Model file for the job. Use its own axes, mm. A direction names the side the tool comes from. Coordinates: 2 decimals unless noted, no trailing zeros. Loops run counter-clockwise (first coordinate to the right, second up) from the corner with the lowest first, then second, coordinate; pieces in that order, holes last. Notation, with made-up numbers: M -0.5,81.5 L 12.5,81.5 A18 cw 12.5,90.5 Z; hole C 60.25,-20.5 d2. An arc over 180 degrees is marked long. Write item = value, one per line. Start each with the question number.
from build123d import *

# Parameters (mm, degrees)
ESQUISSE1_W             = 70
ESQUISSE1_H             = 110
BOSS_EXTRU_1_DEPTH      = 3
ENL_V_MAT_EXTRU_1_DEPTH = 131.418556962
ENL_V_MAT_EXTRU_2_DEPTH = 10


with BuildPart() as part:
    # Esquisse1 → Boss.-Extru.1 (new body)
    with BuildSketch(Plane.XY):
        with Locations((-35, 55)):
            Rectangle(ESQUISSE1_W, ESQUISSE1_H)
    extrude(amount=BOSS_EXTRU_1_DEPTH)

    # Esquisse2 → Enlèv. mat.-Extru.1 (cut, through all)
    with BuildSketch(Plane(origin=(0, 0, 0), x_dir=(-1, 0, 0), z_dir=(0, 0, -1))):
        Polygon((0, 110), (25, 110), (25, 104), (6, 104), (6, 68.5), (0, 68.5), align=None)
        Polygon((70, 110), (45, 110), (45, 104), (64, 104), (64, 68.5), (70, 68.5), align=None)
        Polygon((0, 0), (25, 0), (25, 6), (6, 6), (6, 38.5), (0, 38.5), align=None)
        Polygon((45, 0), (70, 0), (70, 38.5), (64, 38.5), (64, 6), (45, 6), align=None)
    extrude(amount=-ENL_V_MAT_EXTRU_1_DEPTH, mode=Mode.SUBTRACT)

    # Esquisse3 → Enlèv. mat.-Extru.2 (cut)
    with BuildSketch(Plane.XY.offset(3)):
        Polygon((-70, 38.5), (-25, 38.5), (-25, 81.225715449), (-2.235916109, 81.225715449), (-2.235916109, 110), (-25, 110), (-70, 110), align=None)
    extrude(amount=-ENL_V_MAT_EXTRU_2_DEPTH, mode=Mode.SUBTRACT)


solid = part.part
Item 1: Cut at C-C (y = 43.5). Give the cut face in (x, z).
Item 2: 3-axis set-ups, long thin cutter, end or side, ignore diameter. For faces 1 (the flat face through (-45, 38.5, 2)), 2 (the flat face through (-3, 68.5, 1)), 3 (the flat face through (-45, 3, 1)): which of +Z, -Z, +X, -X, +Y, -Y reach the whole face in a straight line?
Item 3: Pin check, flat tips, straight feed: pin 1 Ø1.5 at (y, z) = (17, 1) entering from +X; pin 2 Ø1.5 at (y, z) = (63, 1) entering from +X; pin 3 Ø0.9 at (x, z) = (-11, 1) entering from -Y; pin 4 Ø0.9 at (x, z) = (-51.5, 1.5) entering from +Y. Stop position of each tip, or through.
Item 4: Cut at A-A (z = 1.1). Give the cut face in (x, y), plus the area to 3 significant figures.
Item 5: Cut at B-B (x = -53.5). Give the cut face in (y, z).
Item 6: Probe L1, parallel to Y at x = -34.5, z = 0.35; L2, parallel to X at y = 18.5, z = 1.2; L3, parallel to X at y = 60.5, z = 2.35. List the from-to ranges inside material, lowest first.
Reported:
q1.outline = M -25,0 L 0,0 L 0,3 L -25,3 Z
q2.face_1 = +Z, -Z, -X, +Y
q2.face_2 = +Z, -Z, +X, +Y
q2.face_3 = +Z, -Z, -X, -Y
q3.pin_1 = -6
q3.pin_2 = 0
q3.pin_3 = 6
q3.pin_4 = 38.5
q4.outline = M -64,6 L -45,6 L -45,0 L -25,0 L -25,6 L -6,6 L -6,38.5 L 0,38.5 L 0,68.5 L -6,68.5 L -6,81.23 L -25,81.23 L -25,38.5 L -64,38.5 Z
q4.area = 3,000 mm^2
q5.outline = M 6,0 L 38.5,0 L 38.5,3 L 6,3 Z
q6.L1 = 0 to 38.5
q6.L2 = -64 to -6
q6.L3 = -25 to 0
